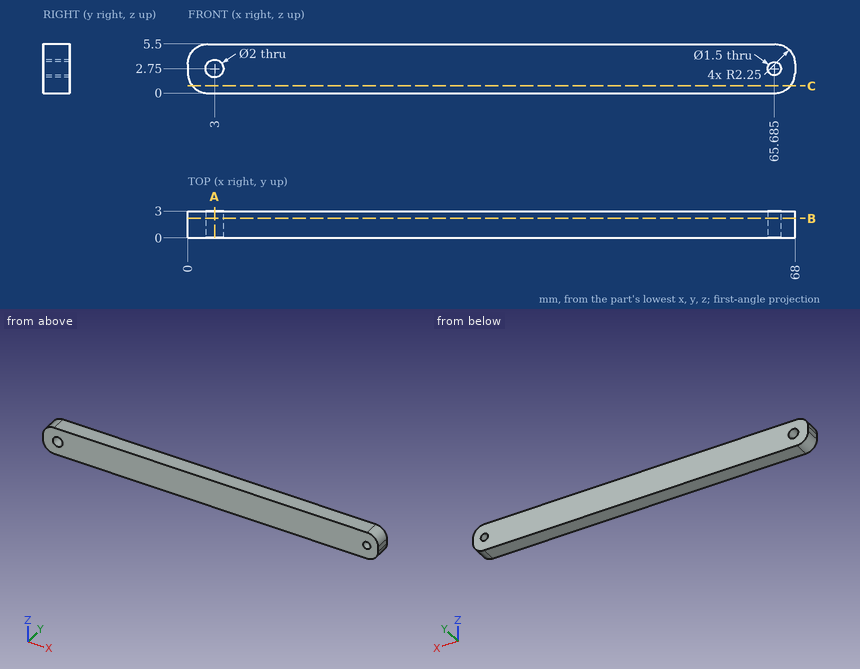
Geometry: see drawing. Coordinates: mm, zero at the bounding-box minimum. Give positions to 0.01 mm unless a question says otherwise; leave off trailing zeros. Order: outer loops, then holes, each group sorted by start corner. A loop starts at its lowest first (then second) coordinate and runs counter-clockwise, first axis right, second up. Notation, with made-up numbers: M 5.5,54.25 L 15.5,54.25 A16 cw 15.5,72.25 Z; hole C 13,54 d1. An arc over 180 degrees is marked long. Answer as a JSON object with one key per item and string values.
1. Cut plane C-C, the plane z = 0.8. Output: boundary loops of the cut face in (x, y), and give its area (3 significant figures).
Result sheet:
{"outline": "M 0.53,0 L 67.47,0 L 67.47,3 L 0.53,3 Z", "area": "201 mm²"}
2. First-contact query: P1, Ø1.6, axis at x = 3, z = 2.75, coming from the +Y side (3 decimals). Flat tip, straight axial feed; report the tip coordinate or a pass-through.
Result sheet:
{"P1": "through"}
3. Ray query, line 1 (X direction, y = 1.65, z = 2.75) (3 decimals); line 2 (X direction, y = 0.3, z = 4.3); line 3 (X direction, y = 0.8, z = 0.6). Return the intervals inside material, ascending. Write a range as [from, to].
Result sheet:
{"line 1": "[0, 2], [4, 64.935], [66.435, 68]", "line 2": "[0.26, 67.74]", "line 3": "[0.72, 67.28]"}
4. Cut plane B-B, the plane y = 2.2. Output: boundary loops of the cut face in (x, z) (3 decimals), and give its area (3 significant figures).
Result sheet:
{"outline": "M 0,2.25 A2.25 ccw 2.25,0 L 65.75,0 A2.25 ccw 68,2.25 L 68,3.25 A2.25 ccw 65.75,5.5 L 2.25,5.5 A2.25 ccw 0,3.25 Z; hole C 3,2.75 d2; hole C 65.685,2.75 d1.5", "area": "365 mm²"}
5. Cut plane A-A, the plane x = 3. Output: boundary loops of the cut face in (y, z), and give its area (3 significant figures).
Result sheet:
{"outline": "M 0,0 L 3,0 L 3,1.75 L 0,1.75 Z; M 0,3.75 L 3,3.75 L 3,5.5 L 0,5.5 Z", "area": "10.5 mm²"}
